The model under review builds one solid part; all positions refer to its coordinate system, in mm. A direction names the side the tool comes from. Give positions to 0.01 mm unless a question says otherwise; leave off trailing zeros. Order: outer loops, then holes, each group sorted by start corner. A loop starts at its lowest first (then second) coordinate and runs counter-clockwise, first axis right, second up.
```python
from build123d import *

# Parameters (mm, degrees)
SKETCH1_W            = 15.9
SKETCH1_H            = 23.85
BOSS_EXTRUDE1_DEPTH  = 15.9
SHELL2_T             = -1.2
SKETCH7_W            = 13.5
SKETCH7_H            = 14.7
BOSS_EXTRUDE4_DEPTH  = 2
SHELL3_START         = -6.75
SHELL3_OUTLINE_W     = 2
SHELL3_OUTLINE_H     = 13.5
SHELL3_DEPTH         = 13.5
BOSS_EXTRUDE3_DEPTH  = 1.2
SKETCH8_W            = 8.5
SKETCH8_H            = 2.8
CUT_EXTRUDE2_DEPTH   = 23.852748741
SKETCH9_W            = 0.5
SKETCH9_H            = 1.4
BOSS_EXTRUDE5_DEPTH  = 12.7
SKETCH10_R           = 3.25
SKETCH10_R_2         = 2.4
BOSS_EXTRUDE6_DEPTH  = 2
SKETCH11_R           = 2.4
SKETCH11_R_2         = 0.9
BOSS_EXTRUDE7_DEPTH  = 1.8
LPATTERN1_COUNT      = 2
LPATTERN1_PITCH      = 8
LPATTERN1_COUNT_DIR2 = 2
LPATTERN1_PITCH_DIR2 = 8


# Read off the part's stored shape, not the designer's step: Shell3
with BuildPart() as part:
    # Sketch1 → Boss-Extrude1 (new body)
    with BuildSketch(Plane.XY):
        Rectangle(SKETCH1_W, SKETCH1_H)
    extrude(amount=-BOSS_EXTRUDE1_DEPTH)

    # Shell2
    shell2_openings = [part.faces().sort_by_distance(p)[0] for p in [
        (0, 0, 0),
    ]]
    offset(amount=SHELL2_T, openings=shell2_openings, kind=Kind.INTERSECTION)

    # Sketch7 → Boss-Extrude4 (add)
    with BuildSketch(Plane(origin=(0, -10.725, 0), x_dir=(1, 0, 0), z_dir=(0, 1, 0))):
        with Locations((0, 7.35)):
            Rectangle(SKETCH7_W, SKETCH7_H)
    extrude(amount=BOSS_EXTRUDE4_DEPTH)

    # Shell3 outline → Shell3 (cut)
    with BuildSketch(Plane.YZ.offset(SHELL3_START)):
        with Locations((-10.925, -7.95)):
            Rectangle(SHELL3_OUTLINE_W, SHELL3_OUTLINE_H)
    extrude(amount=SHELL3_DEPTH, mode=Mode.SUBTRACT)

    # Sketch5 → Boss-Extrude3 (add)
    with BuildSketch(Plane(origin=(6.75, 0, 0), x_dir=(0, 0, -1), z_dir=(1, 0, 0))):
        with BuildLine():
            Line((0, -11.925), (-1.5, -11.925))
            ThreePointArc((-1.5, -11.925), (-3.1, -10.325), (-1.5, -8.725))
            Line((-1.5, -8.725), (0, -8.725))
            Line((0, -8.725), (0, -11.925))
        make_face()
    boss_extrude3 = extrude(amount=-BOSS_EXTRUDE3_DEPTH)

    # Mirror2: Boss-Extrude3 across plane
    add(boss_extrude3.mirror(Plane(origin=(0, 0, 0), x_dir=(0, 0, 1), z_dir=(1, 0, 0))))

    # Sketch8 → Cut-Extrude2 (cut, through all)
    with BuildSketch(Plane.XY.offset(-14.7)):
        with Locations((0, 9.325)):
            Rectangle(SKETCH8_W, SKETCH8_H)
    extrude(amount=-CUT_EXTRUDE2_DEPTH, mode=Mode.SUBTRACT)

    # Sketch9 → Boss-Extrude5 (add)
    with BuildSketch(Plane.XY.offset(-14.7)):
        with Locations((-4.5, 10.025)):
            Rectangle(SKETCH9_W, SKETCH9_H)
    boss_extrude5 = extrude(amount=BOSS_EXTRUDE5_DEPTH)

    # Mirror3: Boss-Extrude5 across plane
    add(boss_extrude5.mirror(Plane(origin=(0, 0, 0), x_dir=(0, 0, 1), z_dir=(1, 0, 0))))

    # Sketch10 → Boss-Extrude6 (add)
    with BuildSketch(Plane.XZ.offset(9.925)):
        with Locations(Location((0, -7.95, 0), (0, 0, 90))):
            Circle(SKETCH10_R)
        with Locations(Location((0, -7.95, 0), (0, 0, 270))):
            Circle(SKETCH10_R_2, mode=Mode.SUBTRACT)
    extrude(amount=BOSS_EXTRUDE6_DEPTH)

    # Sketch11 → Boss-Extrude7 (add)
    with BuildSketch(Plane(origin=(0, 11.925, 0), x_dir=(1, 0, 0), z_dir=(0, 1, 0))):
        with Locations(Location((-4.05, 3.9, 0), (0, 0, 270))):
            Circle(SKETCH11_R)
        with Locations(Location((-4.05, 3.9, 0), (0, 0, 270))):
            Circle(SKETCH11_R_2, mode=Mode.SUBTRACT)
    boss_extrude7 = extrude(amount=BOSS_EXTRUDE7_DEPTH)

    # LPattern1: Boss-Extrude7 2 × 2
    with Locations(*[(i * LPATTERN1_PITCH, 0, -j * LPATTERN1_PITCH_DIR2) for i in range(LPATTERN1_COUNT) for j in range(LPATTERN1_COUNT_DIR2) if (i, j) != (0, 0)]):
        add(boss_extrude7)


solid = part.part
```
1. To check wall thickness, follow line 1 (X direction, y = 13.3, z = -11.9); line 2 (Y direction, x = 5.25, z = -9.75) (3 decimals); line 3 (Y direction, x = -4.5, z = -3) (3 decimals). State the ranges of each line that lie inside material, in increasing order.
2. Draft analysis for pull direction Y (two halves, no side actions). For faces 4 (the cylindrical face through (-4, 13, -11)), 5 (the flat face through (2.9, 13.725, -3.9)), 6 (the flat face through (-4.25, 10, -9)), state which applies: pulls with the +Y half, pulls with the -Y half, needs draft (parallel to the pull), parting line crosses it, or undercut.
3. Take a section at B-B (z = -0.75). Write out the cut boundary in (x, y) (3 decimals), and give its area (3 significant figures).
4. For faces 1 (the flat face through (-6.75, 1, -7)), 2 (the flat face through (-5.55, -10, 2)), 3 (the flat face through (-6.75, -11, -8)), list the 3-axis set-ups (+Z, -Z, +X, -X, +Y, -Y) from which the entire face can be reached by the end or side of a thin tool; tool diameter is ignored.
5. Insertion check: pin 1 (1.6 mm diameter, centred on x = -1.5, y = -10.5, fed in from +Z); pin 2 (7 mm diameter, centred on x = -0.5, z = -10, fed in from +Y) (3 decimals); pin 3 (0.6 mm diameter, centred on x = -4.5, z = -11, fed in from -Y) (3 decimals); pin 4 (2 mm diameter, centred on x = 3, z = -8, fed in from +Y) (3 decimals). Each pin has a flat end and moves straight along its axis. Give the tip position at first contact, or say it passes through.
6. Take a section at D-D (z = -7.95). Write out the cut boundary in (x, y) (3 decimals).
7. Take a section at C-C (y = 1.75). Write out the cut boundary in (x, z).
Answer:
1. line 1: x = -6.45 to -4.95, -3.15 to -1.65, 1.55 to 3.05, 4.85 to 6.35
1. line 2: y = -9.925 to -8.725, 10.725 to 11.925
1. line 3: y = -9.925 to -8.725, 9.325 to 13.725
2. face 4: needs draft
2. face 5: pulls with the +Y half
2. face 6: undercut
3. outline: (-7.95, -11.925) - (7.95, -11.925) - (7.95, 11.925) - (-7.95, 11.925) - close; hole (-6.75, -8.725) - (6.75, -8.725) - (6.75, 10.725) - (-6.75, 10.725) - close
3. area: 117 mm2
4. face 1: +Z
4. face 2: +Z, +Y, -Y
4. face 3: -Y
5. pin 1: stops at z = 0
5. pin 2: stops at y = 13.725
5. pin 3: stops at y = -9.925
5. pin 4: stops at y = 11.925
6. outline: (-7.95, -11.925) - (-6.75, -11.925) - (-6.75, -9.925) - (-3.25, -9.925) - (-3.25, -11.925) - (-2.4, -11.925) - (-2.4, -9.925) - (2.4, -9.925) - (2.4, -11.925) - (3.25, -11.925) - (3.25, -9.925) - (6.75, -9.925) - (6.75, -11.925) - (7.95, -11.925) - (7.95, 11.925) - (-7.95, 11.925) - close; hole (-6.75, -8.725) - (6.75, -8.725) - (6.75, 10.725) - (4.75, 10.725) - (4.75, 9.325) - (4.25, 9.325) - (4.25, 10.725) - (-4.25, 10.725) - (-4.25, 9.325) - (-4.75, 9.325) - (-4.75, 10.725) - (-6.75, 10.725) - close
7. outline: (-7.95, -15.9) - (7.95, -15.9) - (7.95, 0) - (6.75, 0) - (6.75, -14.7) - (-6.75, -14.7) - (-6.75, 0) - (-7.95, 0) - close
